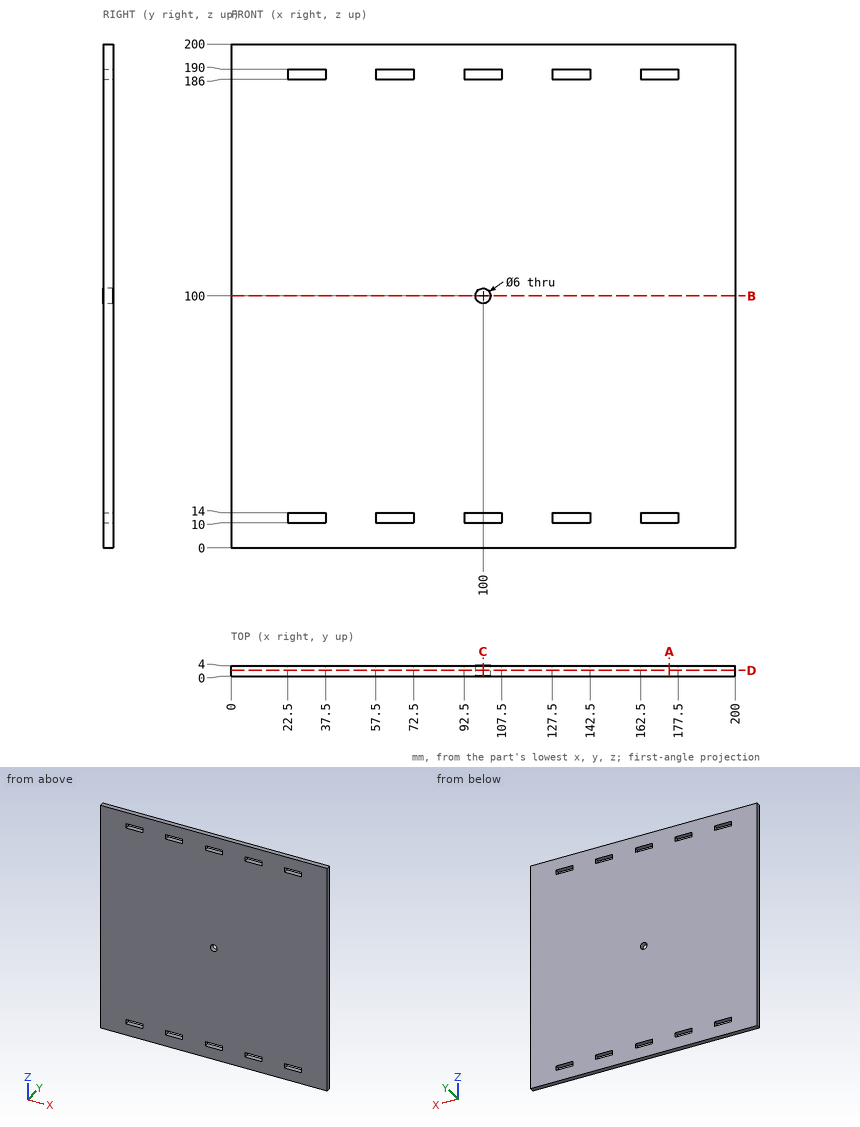
For this review, use the dimensioned drawing (mm, ordinates from the lowest corner) and the shaded views. Give positions to 0.01 mm unless a question says otherwise; leave off trailing zeros. Order: outer loops, then holes, each group sorted by start corner. A loop starts at its lowest first (then second) coordinate and runs counter-clockwise, first axis right, second up.
1) Take a section at A-A (x = 174). Give the boundary of the cut face in (y, z).
2) Wall thickness on line 1 (Z direction, x = 100, y = 1.6); line 2 (Z direction, x = 136, y = 1.1); line 3 (Z direction, x = 99, y = 0.3): over which ranges is each line inside the solid? List them lowest first.
3) Take a section at C-C (x = 100). Give the boundary of the cut face in (y, z), then the cut area to 3 significant figures.
4) Take a section at B-B (z = 100). Give the boundary of the cut face in (x, y), then the cut area to 3 significant figures.
5) Take a section at D-D (y = 2.25). State how many separate pieces and enclosed holes the cut face has, then the cut area to 3 significant figures.
Derived:
1. outline: (0, 0) - (4, 0) - (4, 10) - (0, 10) - close; (0, 14) - (4, 14) - (4, 186) - (0, 186) - close; (0, 190) - (4, 190) - (4, 200) - (0, 200) - close
2. line 1: z = 0 to 10, 14 to 97, 103 to 186, 190 to 200
2. line 2: z = 0 to 10, 14 to 186, 190 to 200
2. line 3: z = 0 to 10, 14 to 97.17, 102.83 to 186, 190 to 200
3. outline: (0, 0) - (4, 0) - (4, 10) - (0, 10) - close; (0, 14) - (4, 14) - (4, 97) - (0, 97) - close; (0, 103) - (4, 103) - (4, 186) - (0, 186) - close; (0, 190) - (4, 190) - (4, 200) - (0, 200) - close
3. area: 744 mm2
4. outline: (0, 0) - (97, 0) - (97, 4) - (0, 4) - close; (103, 0) - (200, 0) - (200, 4) - (103, 4) - close
4. area: 776 mm2
5. separate pieces: 1
5. enclosed holes: 11
5. area: 39,400 mm2
